Part model, mm, in its own coordinate system. Give positions to 0.01 mm unless a question says otherwise; leave off trailing zeros. Order: outer loops, then holes, each group sorted by start corner. A loop starts at its lowest first (then second) coordinate and runs counter-clockwise, first axis right, second up.
1. Drop a flat-ended pin along its axis: pin 1 Ø24 at (x, z) = (25, 0) entering from +Y. Give the stop position or say it passes through.
2. Slice it at B-B on z = 0. List the corners of the cut face in (x, y).
3. Probe line 1 (X direction, y = -11, z = 0.5); line 2 (Z direction, x = 0, y = -12.25); line 3 (Z direction, x = 3, y = -1.25). List the from-to ranges inside material, lowest first.
4. Slice it at D-D on x = 6. List the corners of the cut face in (y, z), and give its area (3 significant figures).
5. Mould opens along X. For faces 1 (the flat face through (-12, 0, 0)), 2 (the cylindrical face through (17.507, -9.86, 0.33)), 3 (the flat face through (-52.5, -10, 0)) say: +X half, -X half, draft (parallel to the pull), parting line (faces both ways), or undercut.
6. Slice it at A-A on x = 25. List the corners of the cut face in (y, z), and give its area (3 significant figures).
7. Slice it at C-C on y = -14.75. List the corners of the cut face in (x, z), and give its area (3 significant figures).
from build123d import *

# Parameters (mm, degrees)
F0_W     = 105
F0_H     = 60
F0_R     = 7.5
F1_DEPTH = 20
F2_R     = 2.5


with BuildPart() as f1:
    # F0 (on Front) → F1 (new body)
    with BuildSketch(Plane.XZ):
        Rectangle(F0_W, F0_H)
        with Locations((-25, 0)):
            Circle(F0_R, mode=Mode.SUBTRACT)
        Circle(F0_R, mode=Mode.SUBTRACT)
        with Locations((25, 0)):
            Circle(F0_R, mode=Mode.SUBTRACT)
    extrude(amount=F1_DEPTH)

    # F2
    f2_edges = [f1.edges().sort_by_distance(p)[0] for p in [
        (0, -20, -30),
        (-52.5, -20, 0),
        (0, -20, 30),
        (52.5, 0, 0),
        (0, 0, -30),
        (-52.5, 0, 0),
        (0, 0, 30),
        (52.5, -20, 0),
    ]]
    fillet(f2_edges, radius=F2_R)


solid = f1.part
Data:
1. pin 1: stops at y = 0
2. outline: (-52.5, -17.5) arc R2.5 ccw to (-50, -20) - (-32.5, -20) - (-32.5, 0) - (-50, 0) arc R2.5 ccw to (-52.5, -2.5) - close; (-17.5, -20) - (-7.5, -20) - (-7.5, 0) - (-17.5, 0) - close; (7.5, -20) - (17.5, -20) - (17.5, 0) - (7.5, 0) - close; (32.5, -20) - (50, -20) arc R2.5 ccw to (52.5, -17.5) - (52.5, -2.5) arc R2.5 ccw to (50, 0) - (32.5, 0) - close
3. line 1: x = -52.5 to -32.48, -17.52 to -7.48, 7.48 to 17.52, 32.48 to 52.5
3. line 2: z = -30 to -7.5, 7.5 to 30
3. line 3: z = -29.67 to -6.87, 6.87 to 29.67
4. outline: (-20, -27.5) arc R2.5 ccw to (-17.5, -30) - (-2.5, -30) arc R2.5 ccw to (0, -27.5) - (0, -4.5) - (-20, -4.5) - close; (-20, 4.5) - (0, 4.5) - (0, 27.5) arc R2.5 ccw to (-2.5, 30) - (-17.5, 30) arc R2.5 ccw to (-20, 27.5) - close
4. area: 1,010 mm2
5. face 1: draft
5. face 2: undercut
5. face 3: -X half
6. outline: (-20, -27.5) arc R2.5 ccw to (-17.5, -30) - (-2.5, -30) arc R2.5 ccw to (0, -27.5) - (0, -7.5) - (-20, -7.5) - close; (-20, 7.5) - (0, 7.5) - (0, 27.5) arc R2.5 ccw to (-2.5, 30) - (-17.5, 30) arc R2.5 ccw to (-20, 27.5) - close
6. area: 895 mm2
7. outline: (-52.5, -30) - (52.5, -30) - (52.5, 30) - (-52.5, 30) - close; hole circle Ø15 at (-25, 0); hole circle Ø15 at (0, 0); hole circle Ø15 at (25, 0)
7. area: 5,770 mm2
